from build123d import *

# Parameters (mm, degrees)
EXTRUDE1_DEPTH     = 3
SKETCH2_R          = 1.5875
EXTRUDE2_DEPTH     = 3
SKETCH3_R          = 1.5875
EXTRUDE3_DEPTH     = 3
SKETCH5_R          = 1.5875
CUT_EXTRUDE1_DEPTH = 3


with BuildPart() as part:
    # Sketch1 → Extrude1 (new body)
    with BuildSketch(Plane(origin=(0, 0, 0), x_dir=(1, 0, 0), z_dir=(0, 1, 0))):
        Polygon((-145, -76), (-22, -76), (-22, -106), (-10, -106), (-10, -96), (0, -96), (0, -10), (-10, -10), (-10, 0), (-135, 0), (-135, -10), (-145, -10), align=None)
    extrude(amount=EXTRUDE1_DEPTH)

    # Sketch2 → Extrude2 (cut)
    with BuildSketch(Plane(origin=(0, 3, 0), x_dir=(1, 0, 0), z_dir=(0, 1, 0))):
        with Locations(Location((-6, -25, 0), (0, 0, 270))):
            Circle(SKETCH2_R)
        with Locations(Location((-6, -82, 0), (0, 0, 270))):
            Circle(SKETCH2_R)
        with Locations(Location((-26.3, -8, 0), (0, 0, 270))):
            Circle(SKETCH2_R)
        with Locations(Location((-124.3, -8, 0), (0, 0, 270))):
            Circle(SKETCH2_R)
    extrude(amount=-EXTRUDE2_DEPTH, mode=Mode.SUBTRACT)

    # Sketch3 → Extrude3 (cut)
    with BuildSketch(Plane(origin=(0, 3, 0), x_dir=(1, 0, 0), z_dir=(0, 1, 0))):
        with Locations(Location((-111, -4, 0), (0, 0, 270))):
            Circle(SKETCH3_R)
        with Locations(Location((-19, -4, 0), (0, 0, 270))):
            Circle(SKETCH3_R)
        with Locations(Location((-43.4, -48.4, 0), (0, 0, 270))):
            Circle(SKETCH3_R)
    extrude(amount=-EXTRUDE3_DEPTH, mode=Mode.SUBTRACT)

    # Sketch5 → Cut-Extrude1 (cut)
    with BuildSketch(Plane(origin=(0, 3, 0), x_dir=(1, 0, 0), z_dir=(0, 1, 0))):
        with Locations(Location((-76.25, -34.5240252, 0), (0, 0, 270))):
            Circle(SKETCH5_R)
    extrude(amount=-CUT_EXTRUDE1_DEPTH, mode=Mode.SUBTRACT)


solid = part.part
Can you work these out from the model? Positions are in its coordinate system, mm. A direction names the side the tool comes from. Give positions to 0.01 mm unless a question says otherwise; leave off trailing zeros. Loops run counter-clockwise (first coordinate to the right, second up) from the corner with the lowest first, then second, coordinate; pieces in that order, holes last. Notation, with made-up numbers: (-9.5, 73.25) -> (22.5, 73.25) arc R21 ccw to (22.5, 105.25) -> close; hole circle Ø8 at (-35.5, -30). An arc over 180 degrees is marked (long way). Return JSON: item names as keys, results as strings.
Q1. I want a section at B-B, the plane z = 8. List the corners of the cut face in (x, y) for me.
Checks:
{"outline": "(-135, 0) -> (-125.89, 0) -> (-125.89, 3) -> (-135, 3) -> close; (-122.71, 0) -> (-27.89, 0) -> (-27.89, 3) -> (-122.71, 3) -> close; (-24.71, 0) -> (-10, 0) -> (-10, 3) -> (-24.71, 3) -> close"}
Q2. I need wall thicknesses on probe 1 along X at (y, z) = (1.05, 4); probe 2 along Z at (x, y) = (-124.3, 1.9); probe 3 along X at (y, z) = (2, 25). Which ranges of each line are inside material? Lowest first, please.
Checks:
{"probe 1": "x = -135 to -112.59, -109.41 to -20.59, -17.41 to -10", "probe 2": "z = 0 to 6.41, 9.59 to 76", "probe 3": "x = -145 to -7.59, -4.41 to 0"}
Q3. I want a section at D-D, the plane y = 0.45. Count the separate pieces of the cut face and the enclosed holes in it, then the cut area to 3 significant figures.
Checks:
{"separate pieces": "1", "enclosed holes": "8", "area": "11,300 mm2"}
Q4. We'd pull the mould along X, two halves only. Please class faces 1 (the face through (-20.55, 1.52, 3.66)), 2 (the face through (-84, 1, 76)), 3 (the face through (-10, 1, 101)): released by +X, released by -X, zero draft, split by the parting line, or undercut.
Checks:
{"face 1": "undercut", "face 2": "zero draft", "face 3": "released by +X"}
Q5. For pin 1 Ø3 at (x, z) = (-6, 25) entering from +Y; pin 2 Ø0.9 at (x, y) = (-83, 1) entering from +Z; pin 3 Ø1.5 at (x, y) = (-5, 2) entering from +Z; pin 4 Ø1.5 at (y, z) = (1, 4.5) entering from +X, each with a flat end and sliding along its axis, tell me the tip position at first contact or that it passes through.
Checks:
{"pin 1": "passes through", "pin 2": "stops at z = 76", "pin 3": "stops at z = 96", "pin 4": "stops at x = -10"}
Q6. On a 3-axis mill with a long thin cutter (end or side, diameter ignored), from which of +Z, -Z, +X, -X, +Y, -Y can I reach the whole of each face in a straight line? I mean faces 4 (the face through (-5, 1, 10)), 5 (the face through (-22, 1, 91)), 6 (the face through (-140, 1, 10)). Say none if no direction works.
Checks:
{"face 4": "-Z, +X, +Y, -Y", "face 5": "+Z, -X, +Y, -Y", "face 6": "-Z, -X, +Y, -Y"}
Q7. I want a section at C-C, the plane x = -6. List the corners of the cut face in (y, z) for me.
Checks:
{"outline": "(0, 10) -> (3, 10) -> (3, 23.41) -> (0, 23.41) -> close; (0, 26.59) -> (3, 26.59) -> (3, 80.41) -> (0, 80.41) -> close; (0, 83.59) -> (3, 83.59) -> (3, 96) -> (0, 96) -> close"}
Q8. I want a section at A-A, the plane x = -111. List the corners of the cut face in (y, z) for me, then the cut area to 3 significant figures.
Checks:
{"outline": "(0, 0) -> (3, 0) -> (3, 2.41) -> (0, 2.41) -> close; (0, 5.59) -> (3, 5.59) -> (3, 76) -> (0, 76) -> close", "area": "218 mm2"}
